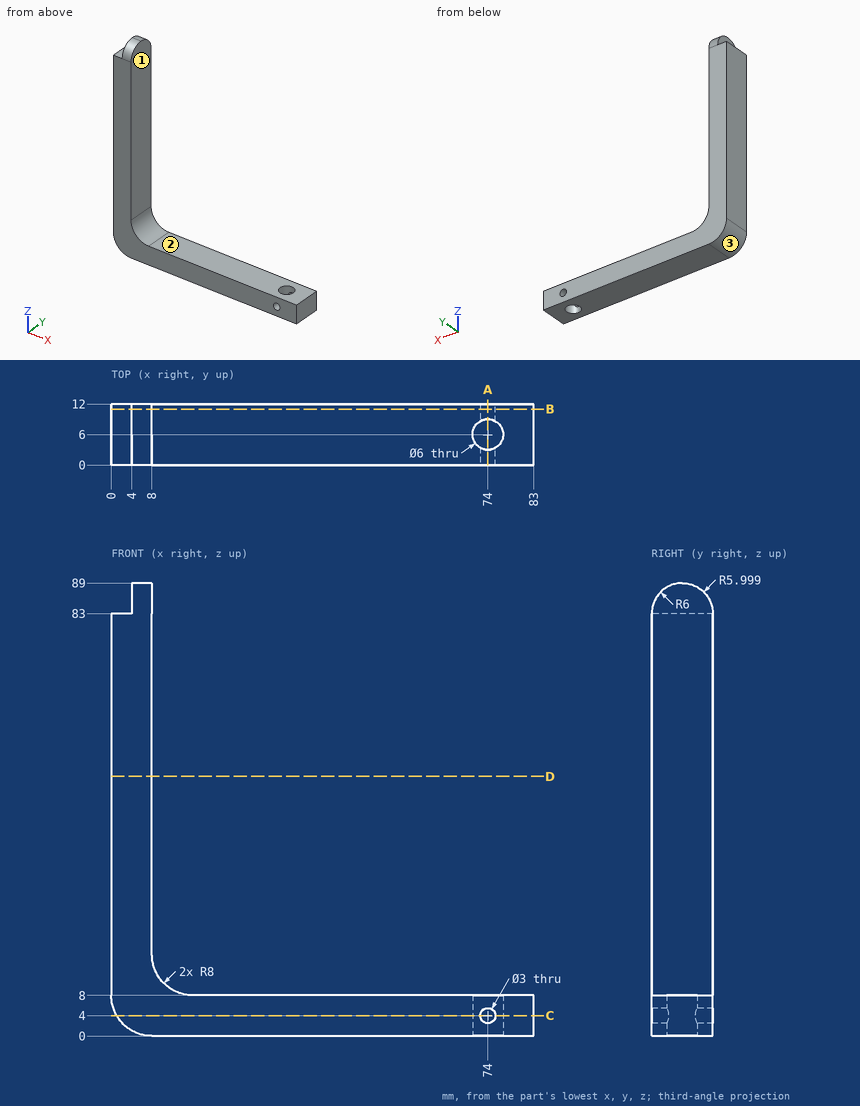
Geometry: see drawing. Coordinates: mm, zero at the bounding-box minimum. Give positions to 0.01 mm unless a question says otherwise; leave off trailing zeros. Loops run counter-clockwise (first coordinate to the right, second up) from the corner with the lowest first, then second, coordinate; pieces in that order, holes last. Notation, with made-up numbers: (44.5, 6.25) -> (69.5, 6.25) arc R19 ccw to (69.5, 29.25) -> close; hole circle Ø2 at (26, 29.25). An arc over 180 degrees is marked (long way). Answer as a JSON object with one key per item and string values. Group by question number.
Item 1: Pin query (flat end, axial travel): P1, Ø3.5, axis at x = 74, y = 6, coming from the -Z side; P2, Ø3.5, axis at y = 5, z = 45, coming from the +X side; P3, Ø6, axis at x = 47.5, y = 4, coming from the +Z side; P4, Ø2, axis at x = 1.5, y = 7, coming from the +Z side. Return the tip coordinate at first contact, or that it passes through.
Item 2: Pull-direction query (Z, two-part tool) for the marked faces 1, 2 and 3; classes: released by +Z, released by -Z, zero draft, split by the parting line, or undercut.
Item 3: Line query: probe 1 along Z at (x, y) = (74, 10.05); probe 2 along Y at (x, z) = (74, 2); probe 3 along Z at (x, y) = (50, 10.75). Output: solid intervals per line, ascending.
Item 4: Cut plane B-B, the plane y = 11. Return the cut outline in (x, z), and give its area (3 significant figures).
Item 5: Cut plane C-C, the plane z = 4. Return the cut outline in (x, y), and give its area (3 significant figures).
Item 6: Cut plane A-A, the plane x = 74. Return the cut outline in (y, z), and give its area (3 significant figures).
Item 7: Cut plane D-D, the plane z = 51. Return the cut outline in (x, y).
Checks:
{
 "1": {"P1": "passes through", "P2": "stops at x = 8", "P3": "stops at z = 8", "P4": "stops at z = 83"},
 "2": {"face 1": "zero draft", "face 2": "released by +Z", "face 3": "released by -Z"},
 "3": {"probe 1": "z = 0 to 2.5, 5.5 to 8", "probe 2": "y = 0 to 3, 9 to 12", "probe 3": "z = 0 to 8"},
 "4": {"outline": "(0, 8) arc R8 ccw to (8, 0) -> (83, 0) -> (83, 8) -> (16, 8) arc R8 cw to (8, 16) -> (8, 86.32) -> (4, 86.32) -> (4, 83) -> (0, 83) -> close; hole circle Ø3 at (74, 4)", "area": "1,270 mm²"},
 "5": {"outline": "(1.07, 0) -> (72.5, 0) -> (72.5, 3.4) arc R3 cw to (72.5, 8.6) -> (72.5, 12) -> (1.07, 12) -> close; (75.5, 0) -> (83, 0) -> (83, 12) -> (75.5, 12) -> (75.5, 8.6) arc R3 cw to (75.5, 3.4) -> close", "area": "936 mm²"},
 "6": {"outline": "(0, 0) -> (3, 0) -> (3, 2.5) -> (0, 2.5) -> close; (0, 5.5) -> (3, 5.5) -> (3, 8) -> (0, 8) -> close; (9, 0) -> (12, 0) -> (12, 2.5) -> (9, 2.5) -> close; (9, 5.5) -> (12, 5.5) -> (12, 8) -> (9, 8) -> close", "area": "30.0 mm²"},
 "7": {"outline": "(0, 0) -> (8, 0) -> (8, 12) -> (0, 12) -> close"}
}
